Geometry: final body of the model. Coordinates: model frame, mm. A direction names the side the tool comes from. Round coordinates to 2 decimals unless told otherwise and drop trailing zeros. Write each loop counter-clockwise with the first axis right and the second up, starting at its lowest first coordinate (ties: lowest second). Pieces come first, ordered by that corner, then holes.
from build123d import *

# Parameters (mm, degrees)
SKETCH2_W           = 5.4034
SKETCH2_H           = 22.6066
SKETCH2_W_2         = 31.9679
SKETCH2_H_2         = 18.2371
BOSS_EXTRUDE1_DEPTH = 3.048
SKETCH3_R           = 1.338245378
CUT_EXTRUDE1_DEPTH  = 4.048
SKETCH4_R           = 1.524
CUT_EXTRUDE2_DEPTH  = 4.048
SKETCH5_W           = 13.7159
SKETCH5_H           = 5.7149
SKETCH5_W_2         = 4.1917
SKETCH5_H_2         = 7.175
CUT_EXTRUDE3_DEPTH  = 4.048
SKETCH7_W           = 12.7
SKETCH7_H           = 1.397
BOSS_EXTRUDE3_DEPTH = 3.048


with BuildPart() as part:
    # Sketch2 → Boss-Extrude1 (new body)
    with BuildSketch(Plane(origin=(0, 0, 8.171752382), x_dir=(-1, 0, 0), z_dir=(0, 0, -1))):
        with BuildLine():
            Line((-23.844892625, -33.084405696), (-34.084892625, -36.451005696))
            ThreePointArc((-34.084892625, -36.451005696), (-36.778969461, -35.335082532), (-37.894892625, -32.641005696))
            Line((-37.894892625, -32.641005696), (-37.894892625, 26.697694304))
            ThreePointArc((-37.894892625, 26.697694304), (-36.778969461, 29.391771141), (-34.084892625, 30.507694304))
            Line((-34.084892625, 30.507694304), (57.404932375, 30.507694304))
            ThreePointArc((57.404932375, 30.507694304), (60.103884597, 29.386886916), (61.214907375, 26.683892153))
            Line((61.214907375, 26.683892153), (61.214907375, 24.068294304))
            Line((61.214907375, 24.068294304), (40.134807375, 24.068294304))
            Line((40.134807375, 24.068294304), (40.134807375, 8.658194304))
            Line((40.134807375, 8.658194304), (56.975007375, 8.658194304))
            Line((56.975007375, 8.658194304), (56.975007375, 4.997894304))
            Line((56.975007375, 4.997894304), (40.134807375, 4.997894304))
            Line((40.134807375, 4.997894304), (40.134807375, -9.121805696))
            Line((40.134807375, -9.121805696), (56.975007375, -9.121805696))
            Line((56.975007375, -9.121805696), (56.975007375, -12.628005696))
            Line((56.975007375, -12.628005696), (35.575007375, -12.628005696))
            Line((35.575007375, -12.628005696), (35.575007375, -28.627805696))
            Line((35.575007375, -28.627805696), (61.214907375, -28.627805696))
            Line((61.214907375, -28.627805696), (61.214907375, -32.613401529))
            ThreePointArc((61.214907375, -32.613401529), (60.108826144, -35.325305244), (57.405007375, -36.451005696))
            Line((57.405007375, -36.451005696), (38.714307375, -36.451005696))
            Line((38.714307375, -36.451005696), (28.474307375, -33.084405696))
            Line((28.474307375, -33.084405696), (28.474307375, -18.034905696))
            Line((28.474307375, -18.034905696), (20.658107375, -18.034905696))
            Line((20.658107375, -18.034905696), (20.658107375, -33.084405696))
            Line((20.658107375, -33.084405696), (10.926407375, -33.084405696))
            Line((10.926407375, -33.084405696), (10.926407375, -20.384405696))
            Line((10.926407375, -20.384405696), (-5.302892625, -20.384405696))
            Line((-5.302892625, -20.384405696), (-5.302892625, -33.084405696))
            Line((-5.302892625, -33.084405696), (-23.844892625, -33.084405696))
        make_face()
        with Locations((16.546707375, -19.663505696)):
            Rectangle(SKETCH2_W, SKETCH2_H, mode=Mode.SUBTRACT)
        Polygon((-29.004892625, -23.698905696), (-22.066892625, -23.698905696), (-22.066892625, -21.185805696), (-19.950892625, -21.185805696), (-19.950892625, -18.920605696), (-17.244692625, -18.920605696), (-17.244692625, -10.792605696), (-23.416892625, -10.792605696), (-23.416892625, 9.801194304), (-29.004892625, 9.801194304), align=None, mode=Mode.SUBTRACT)
        with Locations((-5.654942625, 1.475544304)):
            Rectangle(SKETCH2_W_2, SKETCH2_H_2, mode=Mode.SUBTRACT)
        Polygon((12.361007375, -0.097605696), (17.441007375, -0.097605696), (17.441007375, 15.972394304), (37.825007375, 15.972394304), (37.825007375, 8.658194304), (32.872007375, 8.658194304), (32.872007375, -5.431505696), (12.361007375, -5.431505696), align=None, mode=Mode.SUBTRACT)
        Polygon((0.677107375, 12.372094304), (-29.004794688, 12.372094304), (-29.004892625, 25.896994304), (31.688307375, 25.896994304), (31.688307375, 18.086994304), (0.677107375, 18.086994304), align=None, mode=Mode.SUBTRACT)
    extrude(amount=BOSS_EXTRUDE1_DEPTH)

    # Sketch3 → Cut-Extrude1 (cut, through all)
    with BuildSketch(Plane(origin=(0, 0, 5.123752382), x_dir=(-1, 0, 0), z_dir=(0, 0, -1))):
        with Locations((57.405007375, -32.641005696)):
            Circle(SKETCH3_R)
        with Locations((-34.084892625, -32.641005696)):
            Circle(SKETCH3_R)
        with Locations((-34.084892625, 26.697694304)):
            Circle(SKETCH3_R)
        with Locations((57.404932375, 26.697694304)):
            Circle(SKETCH3_R)
    extrude(amount=-CUT_EXTRUDE1_DEPTH, mode=Mode.SUBTRACT)

    # Sketch4 → Cut-Extrude2 (cut, through all)
    with BuildSketch(Plane(origin=(0, 0, 5.123752382), x_dir=(-1, 0, 0), z_dir=(0, 0, -1))):
        with Locations((-34.084892625, 26.697694304)):
            Circle(SKETCH4_R)
        with Locations((-34.084892625, -32.641005696)):
            Circle(SKETCH4_R)
        with Locations((57.405007375, -32.641005696)):
            Circle(SKETCH4_R)
        with Locations((57.404932375, 26.697694304)):
            Circle(SKETCH4_R)
    extrude(amount=-CUT_EXTRUDE2_DEPTH, mode=Mode.SUBTRACT)

    # Sketch5 → Cut-Extrude3 (cut, through all)
    with BuildSketch(Plane(origin=(0, 0, 5.123752382), x_dir=(-1, 0, 0), z_dir=(0, 0, -1))):
        with Locations((7.535057375, 15.229544304)):
            Rectangle(SKETCH5_W, SKETCH5_H)
        with Locations((33.784157375, 21.674494304)):
            Rectangle(SKETCH5_W_2, SKETCH5_H_2)
    extrude(amount=-CUT_EXTRUDE3_DEPTH, mode=Mode.SUBTRACT)

    # Sketch7 → Boss-Extrude3 (add)
    with BuildSketch(Plane(origin=(0, 0, 5.123752382), x_dir=(-1, 0, 0), z_dir=(0, 0, -1))):
        with Locations((49.175307375, 23.369794304)):
            Rectangle(SKETCH7_W, SKETCH7_H)
    extrude(amount=-BOSS_EXTRUDE3_DEPTH)


solid = part.part
1) Section A-A on x = 4. Output: boundary loops of the cut face in (y, z).
2) Section C-C on x = -52.5. Output: boundary loops of the cut face in (y, z), plus the area to 3 significant figures.
3) Section D-D on y = -16. Output: boundary loops of the cut face in (x, z) (3 decimals).
4) Reachability of faces 1 (the flat face through (-58, 24.068, 7)), 2 (the flat face through (-1, -10, 5.124)), 3 (the flat face through (-25, 18.087, 7)), 4 (the flat face through (-20.658, -25, 7)) from +Z, -Z, +X, -X, +Y, -Y: full face, straight path, thin tool, end or side. Return the list, or none.
5) First-contact query: P1, Ø10, axis at x = -9, y = 20.5, coming from the +Z side; P2, Ø1.1, axis at y = 23, z = 7.5, coming from the -X side; P3, Ø1.5, axis at y = -13, z = 6, coming from the -X side (3 decimals). Flat tips, straight axial feed; report the tip coordinate or a pass-through.
6) Draft query along X for faces 5 (the flat face through (-12.361, -3, 7)), 6 (the flat face through (-17.441, 8, 7)), 7 (the flat face through (-46, -12.628, 7)), 8 (the cylindrical face through (-60.07, 29.42, 6.67)). Return one class per face: pulls with the +X half, pulls with the -X half, needs draft (parallel to the pull), parting line crosses it, or undercut.
7) Line query: probe 1 along Y at (x, z) = (-41.5, 7.2); probe 2 along Y at (x, z) = (-20.5, 5.6); probe 3 along X at (y, z) = (-14.5, 7.8) (3 decimals). Output: solid intervals per line, ascending.
8) Section B-B on y = 6.5. Output: boundary loops of the cut face in (x, z) (3 decimals).
Filled in:
1. outline: (-20.38, 5.12) - (-7.64, 5.12) - (-7.64, 8.17) - (-20.38, 8.17) - close; (10.59, 5.12) - (12.37, 5.12) - (12.37, 8.17) - (10.59, 8.17) - close; (25.9, 5.12) - (30.51, 5.12) - (30.51, 8.17) - (25.9, 8.17) - close
2. outline: (-36.45, 5.12) - (-28.63, 5.12) - (-28.63, 8.17) - (-36.45, 8.17) - close; (-12.63, 5.12) - (-9.12, 5.12) - (-9.12, 8.17) - (-12.63, 8.17) - close; (5, 5.12) - (8.66, 5.12) - (8.66, 8.17) - (5, 8.17) - close; (22.67, 5.12) - (30.51, 5.12) - (30.51, 8.17) - (22.67, 8.17) - close
2. area: 69.6 mm2
3. outline: (-35.575, 5.124) - (-19.248, 5.124) - (-19.248, 8.172) - (-35.575, 8.172) - close; (-13.845, 5.124) - (17.245, 5.124) - (17.245, 8.172) - (-13.845, 8.172) - close; (29.005, 5.124) - (37.895, 5.124) - (37.895, 8.172) - (29.005, 8.172) - close
4. face 1: +Z, -Z, -X
4. face 2: -Z, +X, -X, +Y, -Y
4. face 3: +Z, -Z
4. face 4: +Z, -Z, -Y
5. P1: passes through
5. P2: stops at x = -55.53
5. P3: stops at x = -56.975
6. face 5: undercut
6. face 6: undercut
6. face 7: needs draft
6. face 8: pulls with the -X half
7. probe 1: y = -36.45 to -28.63, -12.63 to -9.12, 5 to 8.66, 24.07 to 30.51
7. probe 2: y = -33.08 to -5.43, 15.97 to 18.09, 25.9 to 30.51
7. probe 3: x = -35.575 to -19.248, -13.845 to 17.245, 29.005 to 37.895
8. outline: (-56.975, 5.124) - (-32.872, 5.124) - (-32.872, 8.172) - (-56.975, 8.172) - close; (-17.441, 5.124) - (-10.329, 5.124) - (-10.329, 8.172) - (-17.441, 8.172) - close; (21.639, 5.124) - (23.417, 5.124) - (23.417, 8.172) - (21.639, 8.172) - close; (29.005, 5.124) - (37.895, 5.124) - (37.895, 8.172) - (29.005, 8.172) - close
